Build history of the part. All positions in model axes, mm. A direction names the side the tool comes from. Coordinates: 2 decimals unless noted, no trailing zeros. One line per item, written item: value.
```python
from build123d import *

# Parameters (mm, degrees)
F0_W     = 139.7
F0_H     = 38.1
F1_DEPTH = 2095.5
F2_R     = 6.35
F3_DEPTH = 152.4
F4_W     = 38.1
F4_H     = 38.1
F5_DEPTH = 44.45


with BuildPart() as f1:
    # F0 (on Top) → F1 (new body)
    with BuildSketch(Plane.XY):
        Rectangle(F0_W, F0_H)
    extrude(amount=F1_DEPTH)

    # F2 (on face) → F3 (cut)
    with BuildSketch(Plane(origin=(-69.85, 0, 0), x_dir=(0, -1, 0), z_dir=(-1, 0, 0))):
        with BuildLine():
            ThreePointArc((6.35, 1047.75), (0, 1054.1), (-6.35, 1047.75))
            Line((-6.35, 1047.75), (6.35, 1047.75))
        make_face()
        with BuildLine():
            Line((6.35, 1047.75), (-6.35, 1047.75))
            ThreePointArc((-6.35, 1047.75), (0, 1041.4), (6.35, 1047.75))
        make_face()
        with Locations((0, 1174.75)):
            Circle(F2_R)
        with Locations((0, 1301.75)):
            Circle(F2_R)
        with Locations((0, 1428.75)):
            Circle(F2_R)
        with Locations((0, 1555.75)):
            Circle(F2_R)
        with Locations((0, 1682.75)):
            Circle(F2_R)
        with Locations((0, 1809.75)):
            Circle(F2_R)
        with Locations((0, 1936.75)):
            Circle(F2_R)
        with Locations((0, 920.75)):
            Circle(F2_R)
        with Locations((0, 666.75)):
            Circle(F2_R)
        with Locations((0, 539.75)):
            Circle(F2_R)
        with Locations((0, 412.75)):
            Circle(F2_R)
        with Locations((0, 285.75)):
            Circle(F2_R)
        with Locations((0, 158.75)):
            Circle(F2_R)
        with Locations((0, 793.75)):
            Circle(F2_R)
        with Locations((0, 2012.95)):
            Circle(F2_R)
        with Locations((0, 82.55)):
            Circle(F2_R)
    extrude(amount=-F3_DEPTH, mode=Mode.SUBTRACT)

    # F4 (on face) → F5 (cut)
    with BuildSketch(Plane.YZ.offset(69.85)):
        with Locations((0, 717.55)):
            Rectangle(F4_W, F4_H)
        with Locations((0, 1377.95)):
            Rectangle(F4_W, F4_H)
    extrude(amount=-F5_DEPTH, mode=Mode.SUBTRACT)


solid = f1.part
```
Item 1: Cut at A-A, the plane x = -12. Give the number of separate pieces and of enclosed holes in the cut face, then the cut area to 3 significant figures.
Check result:
separate pieces: 1
enclosed holes: 17
area: 77,700 mm^2
Item 2: Drop flat-ended pins along their axis: P1, Ø1, axis at y = -1.5, z = 732.5, coming from the +X side; P2, Ø16.5, axis at y = 0, z = 1809.75, coming from the -X side. Give the stop position or say it passes through.
Check result:
P1: stops at x = 25.4
P2: stops at x = -69.85
Item 3: Tool access for faces 1 (the face through (25.4, 0, 718)), 2 (the face through (-1, -19.05, 1033)): list every direction of +Z, -Z, +X, -X, +Y, -Y with a clear straight run to the whole face (end or side of a thin tool).
Check result:
face 1: +X, +Y, -Y
face 2: +Z, -Z, +X, -X, -Y
Item 4: Probe probe 1 along Y at (x, z) = (21.5, 1428.75); probe 2 along Z at (x, y) = (30, 15); probe 3 along X at (y, z) = (-16.5, 731.5). List the from-to ranges inside material, lowest first. Write a range as from..to.
Check result:
probe 1: y = -19.05..-6.35, 6.35..19.05
probe 2: z = 0..698.5, 736.6..1358.9, 1397..2095.5
probe 3: x = -69.85..25.4
Item 5: Pull direction Z, two halves, no side cores. Call faces 3 (the face through (48, 0, 698.5)), 4 (the face through (69.85, 0, 344)), 5 (the face through (-1, 0, 0)): released by +Z, released by -Z, zero draft, split by the parting line, or undercut.
Check result:
face 3: undercut
face 4: zero draft
face 5: released by -Z
